```python
from build123d import *

# Parameters (mm, degrees)
F0_W     = 192
F0_H     = 144
F1_DEPTH = 17
F3_DEPTH = 129.54
F4_R     = 2
F5_R     = 5
F6_R     = 1.5
F7_DEPTH = 3
F6_R_2   = 4.064
F8_DEPTH = 1
F9_DEPTH = 3


with BuildPart() as f1:
    # F0 (on Front) → F1 (new body)
    with BuildSketch(Plane.XZ):
        Rectangle(F0_W, F0_H)
    extrude(amount=F1_DEPTH)

    # F2 (on face) → F3 (join)
    with BuildSketch(Plane(origin=(0, 0, 0), x_dir=(-1, 0, 0), z_dir=(0, 1, 0))):
        with BuildLine():
            ThreePointArc((-92.455, -63.455), (-88.9194660941, -64.9194660941), (-87.455, -68.455))
            Line((-87.455, -68.455), (87.455, -68.455))
            ThreePointArc((87.455, -68.455), (88.9194660941, -64.9194660941), (92.455, -63.455))
            Line((92.455, -63.455), (92.455, 63.455))
            ThreePointArc((92.455, 63.455), (88.9194660941, 64.9194660941), (87.455, 68.455))
            Line((87.455, 68.455), (-87.455, 68.455))
            ThreePointArc((-87.455, 68.455), (-88.9194660941, 64.9194660941), (-92.455, 63.455))
            Line((-92.455, 63.455), (-92.455, -63.455))
        make_face()
    extrude(amount=F3_DEPTH)

    # F4
    f4_edges = [f1.edges().sort_by_distance(p)[0] for p in [
        (-87.455, 64.77, 68.455),
        (-92.455, 64.77, 63.455),
        (-92.455, 64.77, -63.455),
        (-87.455, 64.77, -68.455),
        (87.455, 64.77, -68.455),
        (92.455, 64.77, -63.455),
        (92.455, 64.77, 63.455),
        (87.455, 64.77, 68.455),
    ]]
    fillet(f4_edges, radius=F4_R)

    # F5
    f5_edges = [f1.edges().sort_by_distance(p)[0] for p in [
        (96, -8.5, 72),
        (-96, -8.5, 72),
        (-96, -8.5, -72),
        (96, -8.5, -72),
    ]]
    fillet(f5_edges, radius=F5_R)

    # F6 (on face) → F7 (cut)
    with BuildSketch(Plane(origin=(0, 129.54, 0), x_dir=(-1, 0, 0), z_dir=(0, 1, 0))):
        with Locations((-73.405, 55.755)):
            Circle(F6_R)
        with Locations((-37.337, 55.755)):
            Circle(F6_R)
        with Locations((-13.461, 55.755)):
            Circle(F6_R)
        with Locations((-73.405, 9.781)):
            Circle(F6_R)
        with Locations((-37.337, 9.781)):
            Circle(F6_R)
        with Locations((-13.461, 9.781)):
            Circle(F6_R)
        with Locations((-73.405, -10.285)):
            Circle(F6_R)
        with Locations((-13.461, -56.259)):
            Circle(F6_R)
        with Locations((-37.337, -10.285)):
            Circle(F6_R)
        with Locations((-13.461, -10.285)):
            Circle(F6_R)
        with Locations((-73.405, -56.259)):
            Circle(F6_R)
        with Locations((-37.337, -56.259)):
            Circle(F6_R)
        with Locations((10.413, 46.865)):
            Circle(F6_R)
        with Locations((10.413, 16.385)):
            Circle(F6_R)
        with Locations((58.419, 50.167)):
            Circle(F6_R)
        with Locations((58.419, 0.167)):
            Circle(F6_R)
        with Locations((58.419, -7.745)):
            Circle(F6_R)
        with Locations((58.419, -57.745)):
            Circle(F6_R)
        with Locations((35.813, 1.141)):
            Circle(F6_R)
        with Locations((35.813, -14.353)):
            Circle(F6_R)
    extrude(amount=-F7_DEPTH, mode=Mode.SUBTRACT)

    # F6 (on face) → F8 (join)
    with BuildSketch(Plane(origin=(0, 129.54, 0), x_dir=(-1, 0, 0), z_dir=(0, 1, 0))):
        with Locations((58.955, 58.295)):
            Circle(F6_R_2)
        Polygon((62.0074588497, 59.9328324002), (61.8996338905, 56.4704092923), (58.8471750409, 54.8325768921), (55.9025411503, 56.6571675998), (56.0103661095, 60.1195907077), (59.0628249591, 61.7574231079), align=None, mode=Mode.SUBTRACT)
        Polygon((58.8471750409, 54.8325768921), (61.8996338905, 56.4704092923), (62.0074588497, 59.9328324002), (59.0628249591, 61.7574231079), (56.0103661095, 60.1195907077), (55.9025411503, 56.6571675998), align=None)
    extrude(amount=F8_DEPTH)

    # F6 (on face) → F9 (join)
    with BuildSketch(Plane(origin=(0, 129.54, 0), x_dir=(-1, 0, 0), z_dir=(0, 1, 0))):
        Polygon((58.8471750409, 54.8325768921), (61.8996338905, 56.4704092923), (62.0074588497, 59.9328324002), (59.0628249591, 61.7574231079), (56.0103661095, 60.1195907077), (55.9025411503, 56.6571675998), align=None)
    extrude(amount=F9_DEPTH)


solid = f1.part
```
Work out the finished part from the listing and answer in its coordinate system (mm). A direction names the side the tool comes from. Give positions to 0.01 mm unless a question says otherwise; leave off trailing zeros. Write each loop counter-clockwise with the first axis right and the second up, starting at its lowest first coordinate (ties: lowest second). Pieces come first, ordered by that corner, then holes. Notation, with made-up numbers: (79.5, 89.5) -> (130.5, 89.5) arc R21 cw to (130.5, 117.5) -> close; hole circle Ø2 at (3, 48.5). An arc over 180 degrees is marked (long way). Write each question's results on one line, items separated by ' | '.
1. Each of these flat-tipped pins is pushed along its axis until it touches: pin 1 Ø3.5 at (x, z) = (74, -56.5) entering from +Y; pin 2 Ø0.9 at (x, z) = (73, 10) entering from +Y; pin 3 Ø10 at (x, y) = (31.5, 26.5) entering from -Z (3 decimals). Where does it stop, or does it pass through?
Data:
pin 1: y = 129.54 | pin 2: y = 126.54 | pin 3: z = -68.455
2. Find section A-A on z = 43. Determine the outline of the cut face in (x, y) (3 decimals), and give its area (3 significant figures).
Data:
outline: (-96, -17) -> (96, -17) -> (96, 0) -> (92.455, 0) -> (92.455, 129.54) -> (-92.455, 129.54) -> (-92.455, 0) -> (-96, 0) -> close | area: 27,200 mm^2
3. Straight lines are drawn through the part: L1, parallel to Z at x = -77, y = 33 (3 decimals); L2, parallel to X at y = 3.5, z = 54 (3 decimals); L3, parallel to Y at x = 18.5, z = 16.5. For each, find the intervals that lie inside material, in ascending order.
Data:
L1: -68.455 to 68.455 | L2: -92.455 to 92.455 | L3: -17 to 129.54
4. Find section C-C on y = 19. Determine the outline of the cut face in (x, z) (3 decimals), and give its area (3 significant figures).
Data:
outline: (-92.455, -61.747) arc R2 ccw to (-91.026, -63.663) arc R5 cw to (-87.663, -67.026) arc R2 ccw to (-85.747, -68.455) -> (85.747, -68.455) arc R2 ccw to (87.663, -67.026) arc R5 cw to (91.026, -63.663) arc R2 ccw to (92.455, -61.747) -> (92.455, 61.747) arc R2 ccw to (91.026, 63.663) arc R5 cw to (87.663, 67.026) arc R2 ccw to (85.747, 68.455) -> (-85.747, 68.455) arc R2 ccw to (-87.663, 67.026) arc R5 cw to (-91.026, 63.663) arc R2 ccw to (-92.455, 61.747) -> close | area: 25,200 mm^2
5. A tool of negligible diameter and unlimited length cuts with its end or side. For faces 1 (the flat face through (-1, 64, 68.455)), 2 (the flat face through (-57, 130.54, 61)), 3 (the flat face through (92.455, 64, 1)), 4 (the flat face through (1, 64, -68.455)), 5 (the flat face through (-92.455, 64, -1)), from which of +Z, -Z, +X, -X, +Y, -Y can it reach the whole face along a straight path? Write none if from no direction.
Data:
face 1: +Z, +X, -X, +Y | face 2: +Y | face 3: +Z, -Z, +X, +Y | face 4: -Z, +X, -X, +Y | face 5: +Z, -Z, -X, +Y
6. Find section B-B on x = 68.5. Determine the outline of the cut face in (y, z) (3 decimals), and give its area (3 significant figures).
Data:
outline: (-17, -72) -> (0, -72) -> (0, -68.455) -> (129.54, -68.455) -> (129.54, 68.455) -> (0, 68.455) -> (0, 72) -> (-17, 72) -> close | area: 20,200 mm^2
